```python
from build123d import *

# Parameters (mm, degrees)
PAD_DEPTH    = 20
SKETCH001_R  = 2.25
POCKET_DEPTH = 15.001


with BuildPart() as part:
    # Sketch → Pad (new body)
    with BuildSketch(Plane.XY):
        with BuildLine():
            Line((-17.5, 15), (17.5, 15))
            Line((17.5, 15), (17.5, 0))
            Line((17.5, 0), (6.05, 0))
            ThreePointArc((6.05, 0), (0, 6.05), (-6.05, 0))
            Line((-17.5, 0), (-6.05, 0))
            Line((-17.5, 0), (-17.5, 15))
        make_face()
    extrude(amount=PAD_DEPTH)

    # Sketch001 → Pocket (cut, through all)
    with BuildSketch(Plane.XZ):
        with Locations((-11, 10)):
            Circle(SKETCH001_R)
        with Locations((11, 10)):
            Circle(SKETCH001_R)
    extrude(amount=-POCKET_DEPTH, mode=Mode.SUBTRACT)


solid = part.part
```
Verification items for the finished model (mm, model axes). Give positions to 0.01 mm unless a question says otherwise; leave off trailing zeros. Order: outer loops, then holes, each group sorted by start corner. A loop starts at its lowest first (then second) coordinate and runs counter-clockwise, first axis right, second up. Notation, with made-up numbers: M 8,87.5 L 43,87.5 A35 cw 43,124.5 Z; hole C 21.5,10.25 d9. An arc over 180 degrees is marked long. Return JSON: item names as keys, results as strings. Group by question number.
1) Section check C-C on y = 2.5. Record the cut outline in (x, z), and give its area (3 significant figures).
2) Section check A-A on x = 11. Record the cut outline in (y, z).
3) Section check B-B on z = 10. Record the cut outline in (x, y).
4) Scan lines: line 1 (Z direction, x = 11, y = 5.25); line 2 (X direction, y = 3.25, z = 9); line 3 (Y direction, x = 0, z = 1.5). Record each from-to range of solid material in increasing order.
5) Section check D-D on y = 8.25. Record the cut outline in (x, z).
6) Mould release check, pull along X, two halves, no side actions. Record for faces 1 (the face through (11.9, 0, 7.6)), 2 (the face through (-12.66, 7.4, 11.52)), 3 (the face through (0.13, 6.05, 9.86)), 4 (the face through (-17.5, 7, 10)): pulls with the +X half, pulls with the -X half, needs draft (parallel to the pull), parting line crosses it, or undercut.
7) Go/stop test with flat-tipped pins: pin 1 Ø3 at (x, z) = (3, 15.5) entering from -Y; pin 2 Ø3.5 at (x, z) = (-11, 10) entering from -Y. Record where each tip stops, or that it passes through.
Answer block:
{
 "1": {"outline": "M -17.5,0 L -5.51,0 L -5.51,20 L -17.5,20 Z; M 5.51,0 L 17.5,0 L 17.5,20 L 5.51,20 Z; hole C -11,10 d4.5; hole C 11,10 d4.5", "area": "448 mm^2"},
 "2": {"outline": "M 0,0 L 15,0 L 15,7.75 L 0,7.75 Z; M 0,12.25 L 15,12.25 L 15,20 L 0,20 Z"},
 "3": {"outline": "M -17.5,0 L -13.25,0 L -13.25,15 L -17.5,15 Z; M -8.75,0 L -6.05,0 A6.05 cw 6.05,0 L 8.75,0 L 8.75,15 L -8.75,15 Z; M 13.25,0 L 17.5,0 L 17.5,15 L 13.25,15 Z"},
 "4": {"line 1": "z = 0 to 7.75, 12.25 to 20", "line 2": "x = -17.5 to -13.02, -8.98 to -5.1, 5.1 to 8.98, 13.02 to 17.5", "line 3": "y = 6.05 to 15"},
 "5": {"outline": "M -17.5,0 L 17.5,0 L 17.5,20 L -17.5,20 Z; hole C -11,10 d4.5; hole C 11,10 d4.5"},
 "6": {"face 1": "needs draft", "face 2": "undercut", "face 3": "undercut", "face 4": "pulls with the -X half"},
 "7": {"pin 1": "stops at y = 4.04", "pin 2": "passes through"}
}
